Part model, mm, in its own coordinate system. Round coordinates to 2 decimals unless told otherwise and drop trailing zeros. Write each loop counter-clockwise with the first axis right and the second up, starting at its lowest first coordinate (ties: lowest second). Pieces come first, ordered by that corner, then holes.
from build123d import *

# Parameters (mm, degrees)
SKETCH002_W   = 266
SKETCH002_H   = 166
PAD001_DEPTH  = 4
SKETCH015_W   = 40
SKETCH015_H   = 30
SKETCH015_W_2 = 30
SKETCH015_H_2 = 40
POCKET_DEPTH  = 631.146916
SKETCH034_R   = 3.3
HOLE_DEPTH    = 4.001


with BuildPart() as part:
    # Sketch002 (on DatumPlane) → Pad001 (new body)
    with BuildSketch(Plane(origin=(0, 0, -4), x_dir=(-1, 0, 0), z_dir=(0, 0, 1))):
        Rectangle(SKETCH002_W, SKETCH002_H)
    extrude(amount=-PAD001_DEPTH)

    # Sketch015 (on Face6 of Pad001) → Pocket (cut, through all)
    with BuildSketch(Plane(origin=(0, 0, -8), x_dir=(-1, 0, 0), z_dir=(0, 0, -1))):
        with Locations((-80, 90)):
            Rectangle(SKETCH015_W, SKETCH015_H)
        with Locations((0, 90)):
            Rectangle(SKETCH015_W, SKETCH015_H)
        with Locations((80, 90)):
            Rectangle(SKETCH015_W, SKETCH015_H)
        with Locations((-140, 40)):
            Rectangle(SKETCH015_W_2, SKETCH015_H_2)
        with Locations((-140, -40)):
            Rectangle(SKETCH015_W_2, SKETCH015_H_2)
    pocket = extrude(amount=-POCKET_DEPTH, mode=Mode.SUBTRACT)

    # Mirrored: Pocket across Sketch015 V_Axis
    add(pocket.mirror(Plane(origin=(0, 0, -8), x_dir=(0, 0, -1), z_dir=(-1, 0, 0))), mode=Mode.SUBTRACT)

    # Mirrored001: Pocket across Sketch015 H_Axis
    add(pocket.mirror(Plane(origin=(0, 0, -8), x_dir=(0, 0, -1), z_dir=(0, 1, 0))), mode=Mode.SUBTRACT)

    # Sketch034 (on Face2 of Mirrored001) → Hole (cut, through all)
    with BuildSketch(Plane(origin=(0, 0, -4), x_dir=(-1, 0, 0), z_dir=(0, 0, 1))):
        with Locations((-39.5, 48.5)):
            Circle(SKETCH034_R)
        with Locations((64, 45)):
            Circle(SKETCH034_R)
        with Locations((64, 0)):
            Circle(SKETCH034_R)
        with Locations((-39.5, 3)):
            Circle(SKETCH034_R)
        with Locations((-39.5, -3)):
            Circle(SKETCH034_R)
        with Locations((-39.5, -48.5)):
            Circle(SKETCH034_R)
        with Locations((64, -45)):
            Circle(SKETCH034_R)
        with Locations((110, 60)):
            Circle(SKETCH034_R)
        with Locations((90, 60)):
            Circle(SKETCH034_R)
        with Locations((110, 40)):
            Circle(SKETCH034_R)
        with Locations((90, 40)):
            Circle(SKETCH034_R)
        with Locations((110, 20)):
            Circle(SKETCH034_R)
        with Locations((90, 20)):
            Circle(SKETCH034_R)
        with Locations((110, 0)):
            Circle(SKETCH034_R)
        with Locations((90, 0)):
            Circle(SKETCH034_R)
        with Locations((110, -20)):
            Circle(SKETCH034_R)
        with Locations((90, -20)):
            Circle(SKETCH034_R)
        with Locations((110, -40)):
            Circle(SKETCH034_R)
        with Locations((90, -40)):
            Circle(SKETCH034_R)
        with Locations((110, -60)):
            Circle(SKETCH034_R)
        with Locations((90, -60)):
            Circle(SKETCH034_R)
    extrude(amount=-HOLE_DEPTH, mode=Mode.SUBTRACT)


solid = part.part
Q1. Saw through at C-C, the plane x = 97. Write the cut outline in (y, z), and give its area (3 significant figures).
Q2. Saw through at A-A, the plane x = -110. Give the number of separate pieces and of enclosed holes in the cut face, and give its area (3 significant figures).
Q3. Drop flat-ended pins along their axis: P1, Ø5.5, axis at x = -110, y = -60, coming from the -Z side; P2, Ø2, axis at x = -74.5, z = -5.5, coming from the -Y side. Give the stop position or say it passes through.
Q4. Wall check: line 1 (X direction, y = 48.5, z = -6); line 2 (Y direction, x = -84, z = -4.9); line 3 (X direction, y = -45, z = -5.15). Give the ranges that are in metal, low to high.
Q5. Saw through at B-B, the plane y = 29. Write the cut outline in (x, z), and give its area (3 significant figures).
Q6. Two-plate mould, pull along X, no slides. Class faces 1 (the flat face through (2, -1, -4)), 2 (the cylindrical face through (-106.7, 19.9, -6)): released by +X, released by -X, zero draft, split by the parting line, or undercut.
Computed:
1. outline: (-75, -8) - (75, -8) - (75, -4) - (-75, -4) - close
1. area: 600 mm2
2. separate pieces: 8
2. enclosed holes: 0
2. area: 479 mm2
3. P1: passes through
3. P2: stops at y = -75
4. line 1: x = -125 to 36.2, 42.8 to 125
4. line 2: y = -75 to 75
4. line 3: x = -125 to -67.3, -60.7 to 125
5. outline: (-125, -8) - (125, -8) - (125, -4) - (-125, -4) - close
5. area: 1,000 mm2
6. face 1: zero draft
6. face 2: undercut
